For this review, take the finished solid that the model builds, in its own axes (mm). A direction names the side the tool comes from. Coordinates: 2 decimals unless noted, no trailing zeros. Loops run counter-clockwise (first coordinate to the right, second up) from the corner with the lowest first, then second, coordinate; pieces in that order, holes last. Notation, with made-up numbers: M 77.5,-30.75 L 105.5,-30.75 A37 cw 105.5,7.25 Z; hole C 78.5,12.25 d1. An arc over 180 degrees is marked long. Put each result on its own line as item: value.
Autodesk Inventor part; units mm, degrees
ref_plane "YZ Plane" through (0, 0, 0) normal (1, 0, 0) x (0, 1, 0)
ref_plane "XZ Plane" through (0, 0, 0) normal (0, 1, 0) x (-1, 0, 0)
ref_plane "XY Plane" through (0, 0, 0) normal (0, 0, 1) x (1, 0, 0)
sketch "Sketch1" plane through (0, 0, 0) normal (1, 0, 0) x (0, 1, 0)
  arc A0 (12.7, -17.6415) -> (-12.7, -17.6415) centre (0, -45) ccw
  line L0 (0, 0) -> (0, -134.2841)
  line L1 (-12.7, 0) -> (-12.7, -17.6415)
  line L2 (12.7, -17.6415) -> (12.7, 0)
  line L3 (12.7, 0) -> (-12.7, 0)
  dimension "d0" = 60.325
  dimension "d47" = 45
  dimension "d48" = 25.4
extrude "Extrusion1" add sketch "Sketch1" along normal blind 38.1
sketch "Sketch8" plane through (0, -12.7, 0) normal (0, 0, 1) x (1, 0, 0)
  circle A0 centre (19.05, 12.7) radius 5.05
  line L0 (0, 12.7) -> (38.1, 12.7) construction
  line L1 (0, 25.4) -> (38.1, 25.4) construction
  line L2 (38.1, 25.4) -> (38.1, 0) construction
  dimension "d49" = 10.1
extrude "Extrusion6" cut sketch "Sketch8" against normal through all
sketch "Sketch10" plane through (0, 12.7, 0) normal (0, 1, 0) x (1, 0, 0)
  line L0 (0, 17.6415) -> (0, 0)
  line L1 (0, 0) -> (38.1, 0)
  line L2 (19.05, 0) -> (19.05, 20.4763) construction
  point P0 (19.05, 7.5)
  dimension "d60" = 7.5
hole "Hole2" at (19.05, 12.7, -7.5) direction (0, -1, 0) diameter 5.5 end through all counterbore diameter 10 counterbore depth 4.3
sketch "Sketch11" plane through (0, -12.7, 0) normal (0, 0, 1) x (1, 0, 0)
  line L0 (0, 12.7) -> (38.1, 12.7) construction
  line L1 (38.1, 25.4) -> (38.1, 0) construction
  line L2 (0, 0) -> (38.1, 0) construction
  line L3 (19.05, 0) -> (19.05, 29.1053) construction
  point P0 (31.75, 12.7)
  point P1 (6.35, 12.7)
  dimension "d68" = 25.4
hole "Hole3" at (31.75, 0, 0) at (6.35, 0, 0) direction (0, 0, -1) diameter 5.5 end through all counterbore diameter 9 counterbore depth 4.3
properties part number "Axial Holder" material "ABS Plastic"
(1) Add section C-C (z = -13.25). Write out the cut boundary in (x, y).
Determined:
outline: M 0,-12.7 L 38.1,-12.7 L 38.1,12.7 L 0,12.7 Z; hole C 6.35,0 d5.5; hole C 19.05,0 d10.1; hole C 31.75,0 d5.5
(2) Add section D-D (x = 31.75). Write out the cut boundary in (y, z).
Determined:
outline: M -12.7,-17.64 A30.16 cw -2.75,-14.96 L -2.75,-4.3 L -4.5,-4.3 L -4.5,0 L -12.7,0 Z; M 2.75,-14.96 A30.16 cw 12.7,-17.64 L 12.7,0 L 4.5,0 L 4.5,-4.3 L 2.75,-4.3 Z
(3) Tool access review of faces 5 (the flat face through (34, 2, -4.3)), 6 (the cylindrical face through (20.965, 10.52, -2.881)), 7 (the cylindrical face through (20.7, 6.3, -9.7)): name each direction out of +Z, -Z, +X, -X, +Y, -Y from which nothing blocks a thin tool from reaching the whole face with its end or side.
Determined:
face 5: +Z
face 6: +Y
face 7: +Y, -Y
(4) Add section B-B (x = 19.05). Write out the cut boundary in (y, z), plus the area to 3 significant figures.
Determined:
outline: M -12.7,-17.64 A30.16 cw -5.05,-15.26 L -5.05,-10.25 L -12.7,-10.25 Z; M -12.7,-4.75 L -5.05,-4.75 L -5.05,0 L -12.7,0 Z; M 5.05,-15.26 A30.16 cw 12.7,-17.64 L 12.7,-12.5 L 8.4,-12.5 L 8.4,-10.25 L 5.05,-10.25 Z; M 5.05,-4.75 L 8.4,-4.75 L 8.4,-2.5 L 12.7,-2.5 L 12.7,0 L 5.05,0 Z
area: 145 mm^2
(5) For pin 1 (2.5 mm diameter, centred on x = 33.5, y = 1, fed in from +Z); pin 2 (3 mm diameter, centred on x = 20.5, z = -8.5, fed in from +Y); pin 3 (13 mm diameter, centred on x = 19.05, y = 0, fed in from -Z), all flat-tipped, find the tip position at first contact; note any pin that passes through.
Determined:
pin 1: stops at z = -4.3
pin 2: stops at y = 8.4
pin 3: stops at z = -15.55
(6) Wall thickness on line 1 along X through (y, z) = (0, -8.75); line 2 along X through (y, z) = (0, -3.05); line 3 along X through (y, z) = (-8.5, -7.25): over which ranges is each line inside the solid? List them lowest first. Write a range as [from, to].
Determined:
line 1: x = [0, 3.6], [9.1, 14], [24.1, 29], [34.5, 38.1]
line 2: x = [0, 1.85], [10.85, 14], [24.1, 27.25], [36.25, 38.1]
line 3: x = [0, 16.31], [21.79, 38.1]
(7) Draft analysis for pull direction Y (two halves, no side actions). For faces 1 (the cylindrical face through (36.14, 0.98, -2.18)), 2 (the cylindrical face through (1.89, 0.59, -2.18)), 3 (the flat face through (19, -12.7, -11)), 4 (the flat face through (38.1, 0, -9)), state which applies: +Y half, -Y half, draft (parallel to the pull), parting line (faces both ways), or undercut.
Determined:
face 1: undercut
face 2: undercut
face 3: -Y half
face 4: draft
(8) Add section A-A (z = -7.5). Write out the cut boundary in (x, y).
Determined:
outline: M 0,-12.7 L 16.3,-12.7 L 16.3,-4.24 A5.05 cw 16.3,4.24 L 16.3,8.4 L 14.05,8.4 L 14.05,12.7 L 0,12.7 Z; M 21.8,-12.7 L 38.1,-12.7 L 38.1,12.7 L 24.05,12.7 L 24.05,8.4 L 21.8,8.4 L 21.8,4.24 A5.05 cw 21.8,-4.24 Z; hole C 6.35,0 d5.5; hole C 31.75,0 d5.5
